The model under review builds one solid part; all positions refer to its coordinate system, in mm. Face numbers are marked on the shaded views. Give positions to 0.01 mm unless a question says otherwise; leave off trailing zeros. Loops run counter-clockwise (first coordinate to the right, second up) from the corner with the lowest first, then second, coordinate; pieces in that order, holes last. Notation, with made-up numbers: M -3.75,-25.5 L 28.25,-25.5 A20 ccw 28.25,-10.5 Z; hole C -8.5,1 d1. An arc over 180 degrees is marked long. Write item = value, one per line. Start each with the question number.
1. Wall thickness on line 1 along Z through (x, y) = (4, -34); line 2 along X through (y, z) = (39.5, 88.5); line 3 along Y through (x, z) = (14, 105.5): over which ranges is each line inside the solid? List them lowest first. Write a range as from..to.
2. For pin 1 (12 mm diameter, centred on x = 8, y = -45, fed in from -Z); pin 2 (12 mm diameter, centred on x = -19, z = 118.5, fed in from +Y); pin 3 (4 mm diameter, centred on x = -17.5, y = -22, fed in from -Z); pin 4 (12 mm diameter, centred on x = 2, y = 2, fed in from -Z), all flat-tipped, find the tip position at first contact; note any pin that passes through.
3. Draft analysis for pull direction X (two halves, no side actions). For the marked faces 1 and 2, state which applies: pulls with the +X half, pulls with the -X half, needs draft (parallel to the pull), parting line crosses it, or undercut.
4. We need section A-A on y = 15.5. Give the boundary of the cut face in (x, z), then the cut area to 3 significant figures.
5. We need section B-B on z = 63. Give the boundary of the cut face in (x, y), then the cut area to 3 significant figures.
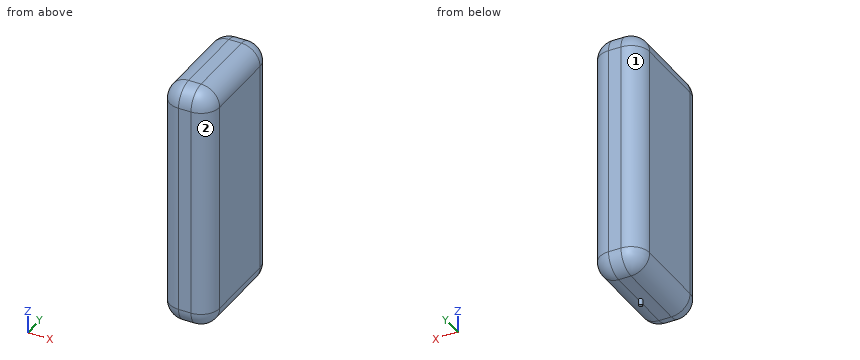
from build123d import *

# Parameters (mm, degrees)
F0_W     = 50.8
F0_H     = 114.3
F1_DEPTH = 254
F2_R     = 1.905
F3_DEPTH = 6.35
F4_F1_R  = 19.05
F4_F2_R  = 19.05
F4_F3_R  = 19.05
F4_F4_R  = 19.05
F4_F5_R  = 19.0499
F4_F6_R  = 19.05


# Not quite as in the source:
# - a fillet or chamfer is up to 0.001 mm smaller than in the source, because OpenCascade refuses the exact size


with BuildPart() as f1:
    # F0 (on Top) → F1 (new body)
    with BuildSketch(Plane.XY):
        Rectangle(F0_W, F0_H)
    extrude(amount=F1_DEPTH)

    # F2 (on face) → F3 (join)
    with BuildSketch(Plane(origin=(0, 0, 0), x_dir=(1, 0, 0), z_dir=(0, 0, -1))):
        with Locations((4.445, 0)):
            Circle(F2_R)
    extrude(amount=F3_DEPTH)

    # F4: fillet of radius 19.05 on 12 edges, made by hand

    # F4_f1
    f4_f1_edges = [f1.edges().sort_by_distance(p)[0] for p in [
        (25.4, -57.15, 127),
    ]]
    fillet(f4_f1_edges, radius=F4_F1_R)

    # F4_f2
    f4_f2_edges = [f1.edges().sort_by_distance(p)[0] for p in [
        (25.4, 57.15, 127),
    ]]
    fillet(f4_f2_edges, radius=F4_F2_R)

    # F4_f3
    f4_f3_edges = [f1.edges().sort_by_distance(p)[0] for p in [
        (-25.4, -57.15, 127),
    ]]
    fillet(f4_f3_edges, radius=F4_F3_R)

    # F4_f4
    f4_f4_edges = [f1.edges().sort_by_distance(p)[0] for p in [
        (-25.4, 57.15, 127),
    ]]
    fillet(f4_f4_edges, radius=F4_F4_R)

    # F4_f5 (radius 19.05 in the source; OpenCascade refuses exactly that, so slightly less here)
    f4_f5_edges = [f1.edges().sort_by_distance(p)[0] for p in [
        (25.4, 0, 0),
    ]]
    fillet(f4_f5_edges, radius=F4_F5_R)

    # F4_f6
    f4_f6_edges = [f1.edges().sort_by_distance(p)[0] for p in [
        (25.4, 0, 254),
    ]]
    fillet(f4_f6_edges, radius=F4_F6_R)


solid = f1.part
Final values:
q1.line_1 = 0..254
q1.line_2 = -25.35..25.35
q1.line_3 = -55.55..55.55
q2.pin_1 = 0.03
q2.pin_2 = 55.95
q2.pin_3 = 2.34
q2.pin_4 = -6.35
q3.face_1 = pulls with the -X half
q3.face_2 = pulls with the +X half
q4.outline = M -25.4,19.05 A19.05 ccw -6.35,0 L 6.35,0 A19.05 ccw 25.4,19.05 L 25.4,234.95 A19.05 ccw 6.35,254 L -6.35,254 A19.05 ccw -25.4,234.95 Z
q4.area = 12,600 mm²
q5.outline = M -25.4,-38.1 A19.05 ccw -6.35,-57.15 L 6.35,-57.15 A19.05 ccw 25.4,-38.1 L 25.4,38.1 A19.05 ccw 6.35,57.15 L -6.35,57.15 A19.05 ccw -25.4,38.1 Z
q5.area = 5,490 mm²
